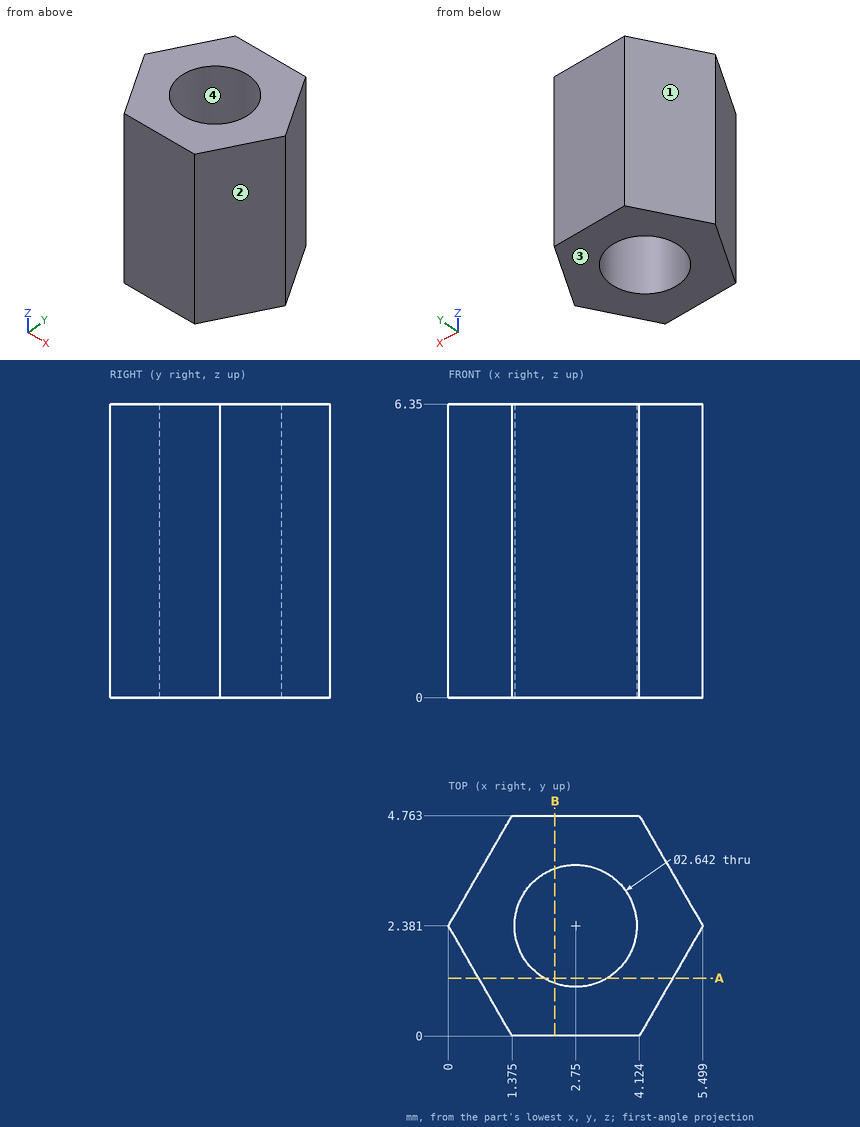
Design review of the part shown in the three views and the two pictorial views. Dimensions are in mm from the part's minimum x, y and z. Give positions to 0.01 mm unless a question says otherwise; leave off trailing zeros. Write each loop counter-clockwise with the first axis right and the second up, starting at its lowest first coordinate (ties: lowest second). Pieces come first, ordered by that corner, then holes. Notation, with made-up numbers: M -14,-29 L 5,-29 A28 ccw 5,0 Z; hole C 37,45.5 d2. An arc over 180 degrees is marked long. One line per question, with ' | ' between items. Start each with the question number.
Item 1: We need section A-A on y = 1.25. Write out the cut boundary in (x, z).
Item 2: For pin 1 (1 mm diameter, centred on y = 3.5, z = 4.5, fed in from +X), flat-tipped, find the tip position at first contact; note if it passes through.
Item 3: We need section B-B on x = 2.3. Write out the cut boundary in (y, z).
Item 4: Draft analysis for pull direction X (two halves, no side actions). For the marked faces 1, 2, 3 and 4, state which applies: released by +X, released by -X, zero draft, split by the parting line, or undercut.
Item 5: Wall thickness on line 1 (Y direction, x = 2.8, z = 4.25); line 2 (Y direction, x = 3.2, z = 4.75); line 3 (X direction, y = 1.7, z = 5.75) (1 decimal): over which ranges is each line inside the solid? List them lowest first. Write a range as from..to.
Results found:
1) outline: M 0.65,0 L 2.07,0 L 2.07,6.35 L 0.65,6.35 Z; M 3.43,0 L 4.85,0 L 4.85,6.35 L 3.43,6.35 Z
2) pin 1: stops at x = 5.14
3) outline: M 0,0 L 1.14,0 L 1.14,6.35 L 0,6.35 Z; M 3.62,0 L 4.76,0 L 4.76,6.35 L 3.62,6.35 Z
4) face 1: released by -X | face 2: released by +X | face 3: zero draft | face 4: undercut
5) line 1: y = 0..1.06, 3.7..4.76 | line 2: y = 0..1.14, 3.62..4.76 | line 3: x = 0.4..1.6, 3.9..5.1
